Build history of the part. All positions in model axes, mm. Face numbers are marked on the shaded views. A direction names the side the tool comes from. Give positions to 0.01 mm unless a question says otherwise; leave off trailing zeros. Loops run counter-clockwise (first coordinate to the right, second up) from the corner with the lowest first, then second, coordinate; pieces in that order, holes last. Notation, with made-up numbers: (-9.5, 75) - (37.5, 75) arc R30 ccw to (37.5, 110) - close; hole circle Ø1 at (71.5, 25). An arc over 180 degrees is marked (long way). Return JSON: item names as keys, results as strings. Group by question number.
1) Slice it at A-A (z = -83.5). List the corners of the cut face in (x, y).
2) Slice it at D-D (z = 141). List the corners of the cut face in (x, y).
3) Mould opens along Z. For the marked faces 4, 5, 6 and 7 say: released by +Z, released by -Z, zero draft, split by the parting line, or undercut.
4) Slice it at C-C (y = 99.5). List the corners of the cut face in (x, z), and give its area (3 significant figures).
5) Drop flat-ended pins along their axis: pin 1 (6 mm diameter, centred on y = 296.5, z = -52.5, fed in from +X); pin 2 (1 mm diameter, centred on y = 329.5, z = -44, fed in from -X); pin 3 (8 mm diameter, centred on x = -129.5, z = 64, fed in from -Y). Give the stop position or say it passes through.
6) Slice it at B-B (x = -15). List the corners of the cut face in (y, z).
7) 3-axis set-ups, long thin cutter, end or side, ignore diameter. For the marked faces 1, 2 and 3: which of +Z, -Z, +X, -X, +Y, -Y reach the whole face in a straight line?
8) Drill centre lines: probe 1 along X at (y, z) = (367, 15.5); probe 2 along Y at (x, z) = (103.5, -167); probe 3 along X at (y, z) = (108.5, -172.5). Where is each one in solid material? Low to high. Write a range as from..to.
```python
from build123d import *

# Parameters (mm, degrees)
IZIM1_R                     = 110
Y_KSEKLIK_EKSTR_ZYON1_DEPTH = 150
Y_KSEKLIK_EKSTR_ZYON2_DEPTH = 850


with BuildPart() as part:
    # Çizim1 → Yükseklik-Ekstrüzyon1 (new body)
    with BuildSketch(Plane(origin=(0, 0, 0), x_dir=(1, 0, 0), z_dir=(0, 1, 0))):
        with BuildLine():
            Line((-45.031937832, 227.98151627), (554.968062168, 227.98151627))
            Line((554.968062168, 227.98151627), (554.968062168, -172.01848373))
            Line((554.968062168, -172.01848373), (-45.031937832, -172.01848373))
            ThreePointArc((-45.031937832, -172.01848373), (-245.031937832, 27.98151627), (-45.031937832, 227.98151627))
        make_face()
        with Locations(Location((-45.031937832, 27.98151627, 0), (0, 0, 270))):
            Circle(IZIM1_R, mode=Mode.SUBTRACT)
    extrude(amount=Y_KSEKLIK_EKSTR_ZYON1_DEPTH)

    # Çizim4 → Yükseklik-Ekstrüzyon2 (add)
    with BuildSketch(Plane(origin=(0, 150, 0), x_dir=(1, 0, 0), z_dir=(0, 1, 0))):
        Polygon((354.968062168, 27.98151627), (354.968062168, 227.98151627), (204.968062168, 227.98151627), (204.968062168, -172.01848373), (354.968062168, -172.01848373), align=None)
    extrude(amount=Y_KSEKLIK_EKSTR_ZYON2_DEPTH)


solid = part.part
```
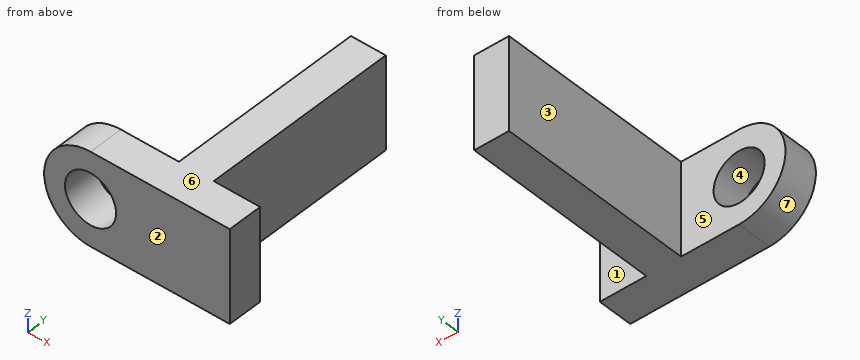
Results:
{
 "1": {"outline": "(-237.17, 0) - (-139.99, 0) - (-139.99, 150) - (-237.17, 150) - close; (49.93, 0) - (554.97, 0) - (554.97, 150) - (354.97, 150) - (354.97, 1000) - (204.97, 1000) - (204.97, 150) - (49.93, 150) - close"},
 "2": {"outline": "(-152.01, 0) - (554.97, 0) - (554.97, 150) - (354.97, 150) - (354.97, 1000) - (204.97, 1000) - (204.97, 150) - (-152.01, 150) - close"},
 "3": {"face 4": "undercut", "face 5": "zero draft", "face 6": "released by +Z", "face 7": "split by the parting line"},
 "4": {"outline": "(-45.03, -227.98) - (554.97, -227.98) - (554.97, 172.02) - (-45.03, 172.02) arc R200 ccw to start; hole circle Ø220 at (-45.03, -27.98)", "area": "265,000 mm2"},
 "5": {"pin 1": "x = 354.97", "pin 2": "x = 204.97", "pin 3": "y = 0"},
 "6": {"outline": "(0, -227.98) - (150, -227.98) - (150, -133.8) - (0, -133.8) - close; (0, 77.84) - (150, 77.84) - (150, 172.02) - (0, 172.02) - close"},
 "7": {"face 1": "+Z, -Z, +X, +Y", "face 2": "+Z, -Z, +X, -X, -Y", "face 3": "+Z, -Z, -X, +Y"},
 "8": {"probe 1": "204.97..354.97", "probe 2": "0..150", "probe 3": "-183.29..554.97"}
}
